from build123d import *

# Parameters (mm, degrees)
SKETCH_1_W             = 40
SKETCH_1_H             = 40
EXTRUDE_1_DEPTH        = 10
SKETCH_2_R             = 10
SKETCH_2_R_2           = 4
EXTRUDE_2_DEPTH        = 5
PATTERN_LINEAR_1_COUNT = 2
PATTERN_LINEAR_1_PITCH = 30


with BuildPart() as part:
    # 草图1 → 凸台-拉伸1 (new body)
    with BuildSketch(Plane.XY):
        Rectangle(SKETCH_1_W, SKETCH_1_H)
    extrude(amount=EXTRUDE_1_DEPTH)

    # 草图2 → 凸台-拉伸2 (add)
    # profile 1 of 2: a face of its own
    with BuildSketch(Plane(origin=(0, 15, 0), x_dir=(1, 0, 0), z_dir=(0, 1, 0))):
        with BuildLine():
            Line((20, -10), (-20, -10))
            Line((-20, -10), (-9.01096744, -32.836181016))
            ThreePointArc((-9.01096744, -32.836181016), (-2.223772201, -18.750392972), (10, -28.5))
            ThreePointArc((10, -28.5), (9.749607028, -30.723772201), (9.01096744, -32.836181016))
            Line((9.01096744, -32.836181016), (20, -10))
        make_face()
    # profile 2 of 2: a face of its own
    with BuildSketch(Plane(origin=(0, 15, 0), x_dir=(1, 0, 0), z_dir=(0, 1, 0))):
        with Locations((0, -28.5)):
            Circle(SKETCH_2_R)
        with Locations(Location((0, -28.5, 0), (0, 0, 270))):
            Circle(SKETCH_2_R_2, mode=Mode.SUBTRACT)
    extrude_2 = extrude(amount=EXTRUDE_2_DEPTH)

    # 阵列(线性)1: 凸台-拉伸2 ×2
    with Locations(*[(0, -i * PATTERN_LINEAR_1_PITCH, 0) for i in range(1, PATTERN_LINEAR_1_COUNT)]):
        add(extrude_2)


solid = part.part
Can you work these out from the model? Positions are in its coordinate system, mm. A direction names the side the tool comes from. Give positions to 0.01 mm unless a question says otherwise; leave off trailing zeros. Loops run counter-clockwise (first coordinate to the right, second up) from the corner with the lowest first, then second, coordinate; pieces in that order, holes last. Notation, with made-up numbers: M 78,67.5 L 84,67.5 A23 ccw 84,85.5 Z; hole C 46.5,63 d3. An arc over 180 degrees is marked long. One line per item, written item: value.
1) Thinking about a two-plate mould opening in X: for faces 4 (the face through (-14.58, -12.54, 21.26)), 5 (the face through (14.429, -12.535, 21.578)), 6 (the face through (-2.4, -12.5, 25.3)), which applies, +X half, -X half, draft (parallel to the pull), parting line (faces both ways), or undercut?
Geometry check:
face 4: -X half
face 5: +X half
face 6: undercut
2) On a 3-axis mill with a long thin cutter (end or side, diameter ignored), from which of +Z, -Z, +X, -X, +Y, -Y can I reach the whole of each face in a straight line? I mean faces 1 (the face through (0, -17, 10)), 2 (the face through (0, 3, 10)), 3 (the face through (-0.2, -12.5, 38.5)). Say none if no direction works.
Geometry check:
face 1: +Z, +X, -X, -Y
face 2: +Z, +X, -X
face 3: +Z, +Y, -Y
3) Imagine slicing it at C-C on z = 21. Write out the boundary of the cut face in (x, y).
Geometry check:
outline: M -14.71,-15 L 14.71,-15 L 14.71,-10 L -14.71,-10 Z; M -14.71,15 L 14.71,15 L 14.71,20 L -14.71,20 Z
4) Imagine slicing it at B-B on z = 28.5. Write out the boundary of the cut face in (x, y).
Geometry check:
outline: M -11.1,-15 L -4,-15 L -4,-10 L -11.1,-10 Z; M -11.1,15 L -4,15 L -4,20 L -11.1,20 Z; M 4,-15 L 11.1,-15 L 11.1,-10 L 4,-10 Z; M 4,15 L 11.1,15 L 11.1,20 L 4,20 Z
5) Please list where these lines run through material, in increasing order: line 1 (Y direction, x = 12, z = 24); line 2 (X direction, y = 16.3, z = 28.5); line 3 (Z direction, x = 17.5, y = 14).
Geometry check:
line 1: y = -15 to -10, 15 to 20
line 2: x = -11.1 to -4, 4 to 11.1
line 3: z = 0 to 10
6) Imagine slicing it at A-A on x = 0. Write out the boundary of the cut face in (y, z), and give its area (3 significant figures).
Geometry check:
outline: M -20,0 L 20,0 L 20,24.5 L 15,24.5 L 15,10 L -10,10 L -10,24.5 L -15,24.5 L -15,10 L -20,10 Z; M -15,32.5 L -10,32.5 L -10,38.5 L -15,38.5 Z; M 15,32.5 L 20,32.5 L 20,38.5 L 15,38.5 Z
area: 605 mm²
7) I'm going to push flat-ended pins straight in: pin 1 (20 mm diameter, centred on x = -4.5, y = 5.5, fed in from +Z); pin 2 (2.5 mm diameter, centred on x = 6.5, y = -18.5, fed in from +Z); pin 3 (23 mm diameter, centred on x = -2.5, z = 24, fed in from -Y). Where does each tip first touch, or does it pass through?
Geometry check:
pin 1: stops at z = 38.4
pin 2: stops at z = 10
pin 3: stops at y = -15
8) Imagine slicing it at D-D on y = 3. Write out the boundary of the cut face in (x, z).
Geometry check:
outline: M -20,0 L 20,0 L 20,10 L -20,10 Z
